Autodesk Inventor part; units mm, degrees
ref_plane "YZ Plane" through (0, 0, 0) normal (1, 0, 0) x (0, 1, 0)
ref_plane "XZ Plane" through (0, 0, 0) normal (0, 1, 0) x (-1, 0, 0)
ref_plane "XY Plane" through (0, 0, 0) normal (0, 0, 1) x (1, 0, 0)
sketch "Sketch1" plane through (0, 0, 0) normal (0, 1, 0) x (-1, 0, 0)
  arc A0 (-22.225, 0) -> (7.3478, 20.9752) centre (0, 0) ccw
  line L0 (-22.225, 0) -> (-12.7, 0)
  line L1 (-12.7, 44.45) -> (-22.225, 44.45)
  line L2 (-22.225, 44.45) -> (-22.225, 0)
  line L3 (39.7917, 0) -> (-48.1139, 0) construction
  line L4 (-10.5747, 27.2537) -> (7.3478, 20.9752)
  line L5 (-12.7, 30.2501) -> (-12.7, 44.45)
  arc A1 (-12.7, 30.2501) -> (-10.5747, 27.2537) centre (-9.525, 30.2501) ccw
  dimension "d0" = 44.45
  dimension "d3" = 9.525
  dimension "d4" = 44.45
  dimension "d5" = 3.175
extrude "Extrusion1" add sketch "Sketch1" along normal blind 25.4
sketch "Sketch2" plane through (0, 25.4, 0) normal (0, 1, 0) x (1, 0, 0)
  circle A0 centre (0, 0) radius 19.05
  dimension "d8" = 38.1
extrude "Extrusion2" cut sketch "Sketch2" against normal blind 20.32
sketch "Sketch3" plane through (0, 5.08, 0) normal (0, 1, 0) x (1, 0, 0)
  circle A0 centre (0, 15.875) radius 1.9844
  circle A1 centre (0, 0) radius 19.05
  circle A2 centre (-13.7482, 7.9375) radius 1.9844
  circle A3 centre (-13.7482, -7.9375) radius 1.9844
  circle A4 centre (0, -15.875) radius 1.9844
  circle A5 centre (13.7482, -7.9375) radius 1.9844
  circle A6 centre (13.7482, 7.9375) radius 1.9844
  circle A7 centre (0, 0) radius 13.4938
  point P0 (0, 0)
  point P1 (0, 19.05)
  dimension "d11" = 3.9688
  dimension "d12" = 3.175
  dimension "d15" = 360
  dimension "d17" = 5.5563
extrude "Extrusion3" cut sketch "Sketch3" against normal up to next contours A0 | A2 | A3 | A4 | A5 | A6 | A7
sketch "Sketch5" plane through (0, 25.4, 0) normal (0, 1, 0) x (1, 0, 0)
  circle A0 centre (0, 0) radius 19.05
  line L0 (12.7, -44.45) -> (22.225, -44.45)
  line L1 (22.225, -44.45) -> (22.225, 0)
  arc A1 (22.225, 0) -> (-7.3478, -20.9752) centre (0, 0) ccw
  line L2 (-7.3478, -20.9752) -> (10.5747, -27.2537)
  arc A2 (12.7, -30.2501) -> (10.5747, -27.2537) centre (9.525, -30.2501) ccw
  line L3 (12.7, -30.2501) -> (12.7, -44.45)
extrude "Extrusion5" add sketch "Sketch5" along normal blind 7.62
sketch "Sketch4" plane through (12.7, 0, 30.2501) normal (-1, 0, 0) x (0, 0, 1)
  circle A0 centre (7.0999, 26.67) radius 1.8034
  line L0 (0, 0) -> (0, 25.4) construction
  line L1 (0, 24.4432) -> (14.1999, 24.4432) construction
  line L2 (14.1999, 24.4432) -> (7.0999, 24.4432) construction
  line L3 (7.0999, 24.4432) -> (7.0999, 0) construction
  line L4 (14.1999, 0) -> (-30.2501, 0) construction
  circle A1 centre (7.0999, 16.51) radius 1.8034
  circle A2 centre (7.0999, 6.35) radius 1.8034
  line L5 (14.1999, 0) -> (14.1999, 33.02)
  line L6 (14.1999, 16.51) -> (0, 16.51) construction
  dimension "d20" = 3.6068
  dimension "d21" = 3.6068
  dimension "d22" = 3.6068
  dimension "d23" = 10.16
  dimension "d24" = 10.16
extrude "Extrusion4" cut sketch "Sketch4" against normal up to next
properties part number "MotorMountA"
Read the model definition and answer for the solid it produces. Units are mm, in the model's axes. A direction names the side the tool comes from. Give positions to 0.01 mm unless a question says otherwise; leave off trailing zeros. Loops run counter-clockwise (first coordinate to the right, second up) from the corner with the lowest first, then second, coordinate; pieces in that order, holes last. Notation, with made-up numbers: (-23, 88.5) -> (-5, 88.5) arc R25 cw to (-5, 126.5) -> close; hole circle Ø4 at (57, -32.75). An arc over 180 degrees is marked (long way). Answer as CSV lines item,"result".
Item 1: For faces 1 (the face through (-12.8, 5.08, 5.6)), 2 (the face through (17.4, 4.59, 36.96)), determine the directions among +Z, -Z, +X, -X, +Y, -Y from which every point of the face is accessible in a straight line to the end or side of a thin tool.
Returned:
face 1,"+Y"
face 2,"+X, -X"
Item 2: Consider line 1 (X direction, y = 1.75, z = 0) (3 decimals); line 2 (Z direction, x = 0, y = 3.5) (3 decimals); line 3 (Y direction, x = 17, z = 37). Determine where each line is inside the solid, lowest interval first. Write a range as [from, to].
Returned:
line 1,"x = [-22.225, -13.494], [13.494, 22.225]"
line 2,"z = [-22.225, -17.859], [-13.891, -13.494], [13.494, 13.891], [17.859, 23.549]"
line 3,"y = [0, 4.58], [8.12, 14.74], [18.28, 24.9], [28.44, 33.02]"
Item 3: Determine the mould class of faces 3 (the face through (13, 33.02, 16)), 4 (the face through (12.7, 16, 34)), 5 (the face through (0.916, 2.576, -14.114)), 6 (the face through (22.225, 16, 23)) for opening direction X: +X half, -X half, draft (parallel to the pull), parting line (faces both ways), or undercut.
Returned:
face 3,"draft"
face 4,"-X half"
face 5,"undercut"
face 6,"+X half"
Item 4: Find section C-C on x = 7. Give the vertices of the cut face in (y, z).
Returned:
outline,"(0, -21.09) -> (33.02, -21.09) -> (33.02, -17.72) -> (5.08, -17.72) -> (5.08, -11.54) -> (0, -11.54) -> close; (0, 11.54) -> (5.08, 11.54) -> (5.08, 17.72) -> (33.02, 17.72) -> (33.02, 26) -> (0, 26) -> close"
Item 5: Find section B-B on y = 16.51. Give the vertices of the cut face in (x, z) (3 decimals).
Returned:
outline,"(-7.348, 20.975) arc R22.225 ccw (long way) to (22.225, 0) -> (22.225, 35.547) -> (12.7, 35.547) -> (12.7, 30.25) arc R3.175 cw to (10.575, 27.254) -> close; (12.7, 39.153) -> (22.225, 39.153) -> (22.225, 44.45) -> (12.7, 44.45) -> close; hole circle Ø38.1 at (0, 0)"
Item 6: Find section A-A on z = 37.35. Give the vertices of the cut face in (x, y) (3 decimals), plus the area to 3 significant figures.
Returned:
outline,"(12.7, 0) -> (22.225, 0) -> (22.225, 4.547) -> (12.7, 4.547) -> close; (12.7, 8.153) -> (22.225, 8.153) -> (22.225, 14.707) -> (12.7, 14.707) -> close; (12.7, 18.313) -> (22.225, 18.313) -> (22.225, 24.867) -> (12.7, 24.867) -> close; (12.7, 28.473) -> (22.225, 28.473) -> (22.225, 33.02) -> (12.7, 33.02) -> close"
area,"211 mm²"
Item 7: Each of these flat-tipped pins is pushed along its axis until it touches: pin 1 (1.5 mm diameter, centred on x = 15.5, z = -7, fed in from +Y); pin 2 (1 mm diameter, centred on y = 6, z = -15.5, fed in from +X); pin 3 (3 mm diameter, centred on x = -4, y = 22, fed in from +Z). Where does it stop, or does it pass through?
Returned:
pin 1,"stops at y = 5.08"
pin 2,"stops at x = 16.4"
pin 3,"stops at z = 22.67"
Item 8: Find section D-D on y = 13. Give the vertices of the cut face in (x, z) (3 decimals), plus the area to 3 significant figures.
Returned:
outline,"(-7.348, 20.975) arc R22.225 ccw (long way) to (22.225, 0) -> (22.225, 44.45) -> (12.7, 44.45) -> (12.7, 30.25) arc R3.175 cw to (10.575, 27.254) -> close; hole circle Ø38.1 at (0, 0)"
area,"779 mm²"
